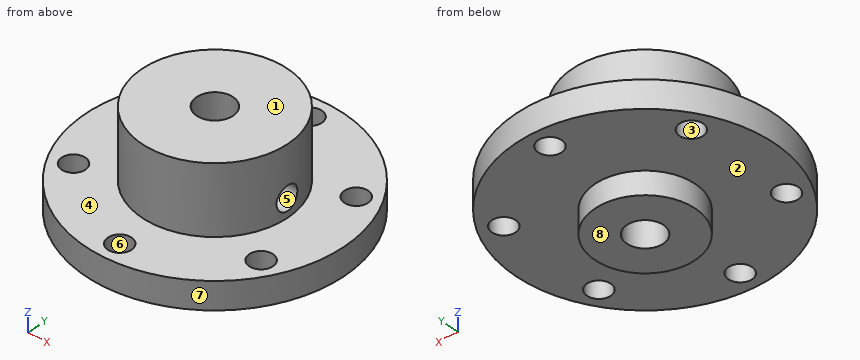
from build123d import *

# Parameters (mm, degrees)
SKETCH_1_R               = 28.35
EXTRUDE_1_DEPTH          = 6
SKETCH_2_R               = 16
EXTRUDE_2_DEPTH          = 15
SKETCH_7_R               = 11
EXTRUDE_3_DEPTH          = 5
SKETCH_3_R               = 4
CUT_EXTRUDE_1_DEPTH      = 27
SKETCH_4_R               = 2.6
CUT_EXTRUDE_2_DEPTH      = 6
PATTERN_CIRCULAR_1_COUNT = 6
CUT_EXTRUDE_3_REACH      = 46.35
SKETCH_6_R               = 2.6


with BuildPart() as part:
    # Sketch 1 → Extrude 1 (new body)
    with BuildSketch(Plane.XY):
        Circle(SKETCH_1_R)
    extrude(amount=EXTRUDE_1_DEPTH)

    # Sketch 2 → Extrude 2 (add)
    with BuildSketch(Plane.XY.offset(6)):
        Circle(SKETCH_2_R)
    extrude(amount=EXTRUDE_2_DEPTH)

    # Sketch 7 → Extrude 3 (add)
    with BuildSketch(Plane(origin=(0, 0, 0), x_dir=(-1, 0, 0), z_dir=(0, 0, -1))):
        Circle(SKETCH_7_R)
    extrude(amount=EXTRUDE_3_DEPTH)

    # Sketch 3 → Cut-Extrude 1 (cut, through all)
    with BuildSketch(Plane.XY.offset(21)):
        Circle(SKETCH_3_R)
    extrude(amount=-CUT_EXTRUDE_1_DEPTH, mode=Mode.SUBTRACT)

    # Sketch 4 → Cut-Extrude 2 (cut)
    with BuildSketch(Plane.XY.offset(6)):
        with Locations((0, 23.75)):
            Circle(SKETCH_4_R)
    cut_extrude_2 = extrude(amount=-CUT_EXTRUDE_2_DEPTH, mode=Mode.SUBTRACT)

    # Pattern Circular 1: Cut-Extrude 2 ×6 about axis
    pattern_circular_1_axis = Axis((0, 0, 0), (0, 0, 1))
    for i in range(1, PATTERN_CIRCULAR_1_COUNT):
        add(cut_extrude_2.rotate(pattern_circular_1_axis, i * 360 / PATTERN_CIRCULAR_1_COUNT), mode=Mode.SUBTRACT)

    # Sketch 6 → Cut-Extrude 3 (cut, up to next)
    with BuildSketch(Plane(origin=(16, 0, 0), x_dir=(0, 0, -1), z_dir=(1, 0, 0)), mode=Mode.PRIVATE) as cut_extrude_3_sk1:
        with Locations((-10, 0)):
            Circle(SKETCH_6_R)
    cut_extrude_3_tool1 = extrude(cut_extrude_3_sk1.sketch, amount=-CUT_EXTRUDE_3_REACH, mode=Mode.PRIVATE) & part.part
    add(cut_extrude_3_tool1.solids().sort_by_distance((16, 0, 10))[0], mode=Mode.SUBTRACT)


solid = part.part
Here's how the part is built. I have some questions about the finished solid (model axes, mm). Face numbers are marked on the shaded views. A direction names the side the tool comes from. Coordinates: 2 decimals unless noted, no trailing zeros. Loops run counter-clockwise (first coordinate to the right, second up) from the corner with the lowest first, then second, coordinate; pieces in that order, holes last.
1. Imagine slicing it at C-C, the plane y = 13. Please give me the cut outline in (x, z).
2. Imagine slicing it at B-B, the plane y = -23.75. Please give me the cut outline in (x, z), and give its area (3 significant figures).
3. For the marked faces 1, 2, 3, 4 and 5, which set-ups out of +Z, -Z, +X, -X, +Y, -Y let a thin tool reach every point of the face, with its end or its side?
4. Imagine slicing it at D-D, the plane z = 1.25. Please give me the cut outline in (x, y) (3 decimals), and give its area (3 significant figures).
5. For P1, Ø1.5, axis at y = 12.5, z = 2, coming from the -X side; P2, Ø6, axis at x = 0, y = -23.75, coming from the +Z side; P3, Ø6, axis at y = 0, z = 10, coming from the +X side; P4, Ø9, axis at x = 0, y = 0, coming from the +Z side, each with a flat end and sliding along its axis, tell me the tip position at first contact or that it passes through.
6. Imagine slicing it at A-A, the plane x = 0. Please give me the cut outline in (y, z).
7. I need wall thicknesses on L1, parallel to Y at x = 0, z = 2.95; L2, parallel to Z at x = 24, y = -14; L3, parallel to Z at x = 11, y = 3.5. Which ranges of each line are inside material? Lowest first, please.
8. If we mould it in two halves opening along X, with no side actions, what happens to the marked faces 6, 7 and 8? For each: pulls with the +X half, pulls with the -X half, needs draft (parallel to the pull), parting line crosses it, or undercut.
Taken from the geometry:
1. outline: (-25.19, 0) - (-22.91, 0) - (-22.91, 6) - (-25.19, 6) - close; (-18.22, 0) - (18.22, 0) - (18.22, 6) - (9.33, 6) - (9.33, 21) - (-9.33, 21) - (-9.33, 6) - (-18.22, 6) - close; (22.91, 0) - (25.19, 0) - (25.19, 6) - (22.91, 6) - close
2. outline: (-15.48, 0) - (-2.6, 0) - (-2.6, 6) - (-15.48, 6) - close; (2.6, 0) - (15.48, 0) - (15.48, 6) - (2.6, 6) - close
2. area: 155 mm2
3. face 1: +Z, +X, -X, +Y, -Y
3. face 2: -Z
3. face 3: +Z, -Z
3. face 4: +Z
3. face 5: +X
4. outline: circle Ø56.7 at (0, 0); hole circle Ø5.2 at (-20.568, -11.875); hole circle Ø5.2 at (-20.568, 11.875); hole circle Ø8 at (0, 0); hole circle Ø5.2 at (0, -23.75); hole circle Ø5.2 at (0, 23.75); hole circle Ø5.2 at (20.568, -11.875); hole circle Ø5.2 at (20.568, 11.875)
4. area: 2,350 mm2
5. P1: stops at x = -25.8
5. P2: stops at z = 6
5. P3: stops at x = 16
5. P4: stops at z = 21
6. outline: (-28.35, 0) - (-26.35, 0) - (-26.35, 6) - (-28.35, 6) - close; (-21.15, 0) - (-11, 0) - (-11, -5) - (-4, -5) - (-4, 21) - (-16, 21) - (-16, 6) - (-21.15, 6) - close; (4, -5) - (11, -5) - (11, 0) - (21.15, 0) - (21.15, 6) - (16, 6) - (16, 21) - (4, 21) - close; (26.35, 0) - (28.35, 0) - (28.35, 6) - (26.35, 6) - close
7. L1: y = -28.35 to -26.35, -21.15 to -4, 4 to 21.15, 26.35 to 28.35
7. L2: z = 0 to 6
7. L3: z = 0 to 21
8. face 6: undercut
8. face 7: parting line crosses it
8. face 8: needs draft
